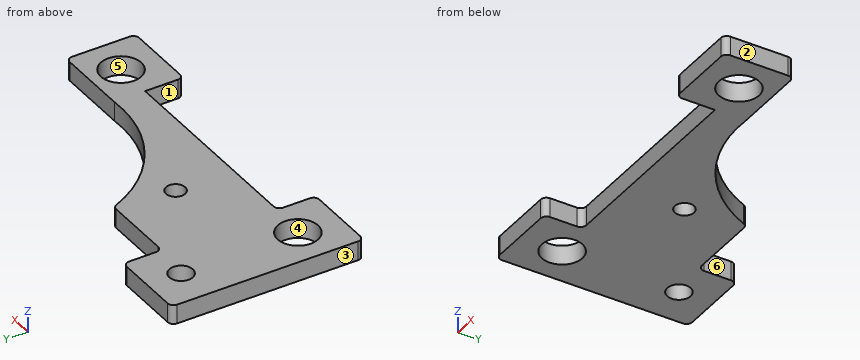
Autodesk Inventor part; units mm, degrees
ref_plane "YZ Plane" through (0, 0, 0) normal (1, 0, 0) x (0, 1, 0)
ref_plane "XZ Plane" through (0, 0, 0) normal (0, 1, 0) x (-1, 0, 0)
ref_plane "XY Plane" through (0, 0, 0) normal (0, 0, 1) x (1, 0, 0)
sketch "Esboço1" plane through (0, 0, 0) normal (0, 1, 0) x (-1, 0, 0)
  point P0 (0, 0)
sketch "Esboço2" plane through (0, 0, 0) normal (0, 0, 1) x (1, 0, 0)
  line L0 (0, 0) -> (20, 0)
  line L1 (20, 0) -> (20, 10)
  line L2 (20, 10) -> (75, 10)
  line L3 (75, 10) -> (75, 0)
  line L4 (75, 0) -> (95, 0)
  line L5 (95, 0) -> (95, 18)
  line L6 (95, 18) -> (75, 18)
  line L7 (0, 0) -> (0, 50)
  line L8 (0, 50) -> (20, 50)
  line L9 (20, 50) -> (20, 40)
  line L10 (20, 40) -> (40, 40)
  arc A0 (40, 40) -> (75, 18) centre (72.5309, 52.9128) ccw
  circle A1 centre (10, 41.2323) radius 3.05
  circle A2 centre (10, 10.8785) radius 5.25
  circle A3 centre (85, 10) radius 5.25
  circle A4 centre (38.286, 25) radius 2.5
  dimension "d0" = 20
  dimension "d1" = 10
  dimension "d2" = 55
  dimension "d3" = 10
  dimension "d4" = 20
  dimension "d5" = 18
  dimension "d6" = 20
  dimension "d7" = 50
  dimension "d8" = 20
  dimension "d9" = 10
  dimension "d10" = 20
  dimension "d11" = 35
  dimension "d12" = 6.1
  dimension "d13" = 10.5
  dimension "d14" = 10.5
  dimension "d15" = 5
extrude "Extrusão1" add sketch "Esboço2" along normal blind 5
fillet "Arredondamento1" radius 1.5 2 edges at (0, 50, 2.5) (20, 50, 2.5)
fillet "Arredondamento2" radius 1.5 8 edges at (20, 40, 2.5) (40, 40, 2.5) (95, 0, 2.5) (75, 0, 2.5) (20, 0, 2.5) (20, 10, 2.5) (95, 18, 2.5) (0, 0, 2.5)
properties part number "lateralCanhao"
Check sheet for the modelled part. Datum: model origin and axes. Units: mm. Face numbers are marked on the shaded views. A direction names the side the tool comes from. Round coordinates to 2 decimals unless told otherwise and drop trailing zeros. Order: outer loops, then holes, each group sorted by start corner. A loop starts at its lowest first (then second) coordinate and runs counter-clockwise, first axis right, second up.
(1) Go/stop test with flat-tipped pins: P1, Ø17, axis at x = 85, y = 10, coming from the -Z side; P2, Ø3, axis at x = 38.286, y = 25, coming from the +Z side; P3, Ø2.5, axis at x = 82, z = 1.5, coming from the +Y side; P4, Ø2.5, axis at x = 42, z = 1.5, coming from the -Y side. Record where each tip stops, or that it passes through.
(2) Draft check along X on the marked faces 3, 4, 5 and 6. Enter one of: pulls with the +X half, pulls with the -X half, needs draft (parallel to the pull), parting line crosses it, or undercut.
(3) Cross-section at B-B, the plane x = 85. Enter the section's corners in (y, z).
(4) Cross-section at D-D, the plane y = 25. Enter the section's corners in (x, z), and give its area (3 significant figures).
(5) Cross-section at C-C, the plane z = 2.1. Enter the section's corners in (x, y), and give its area (3 significant figures).
(6) Scan lines: probe 1 along Y at (x, z) = (10, 1.45); probe 2 along Y at (x, z) = (85, 3.3); probe 3 along X at (y, z) = (11.5, 4.55). Record each from-to range of solid material in increasing order.
(7) Cross-section at A-A, the plane x = 10. Enter the section's corners in (y, z), and give its area (3 significant figures).
(8) Access from +Z, -Z, +X, -X, +Y, -Y to the whole of each face (thin tool, end or side, straight path). Record for the marked faces 1 and 2.
Check sheet entries:
1. P1: stops at z = 0
1. P2: passes through
1. P3: stops at y = 18
1. P4: stops at y = 10
2. face 3: pulls with the -X half
2. face 4: undercut
2. face 5: undercut
2. face 6: pulls with the +X half
3. outline: (0, 0) - (4.75, 0) - (4.75, 5) - (0, 5) - close; (15.25, 0) - (18, 0) - (18, 5) - (15.25, 5) - close
4. outline: (0, 0) - (35.79, 0) - (35.79, 5) - (0, 5) - close; (40.79, 0) - (51.42, 0) - (51.42, 5) - (40.79, 5) - close
4. area: 232 mm2
5. outline: (0, 1.5) arc R1.5 ccw to (1.5, 0) - (18.5, 0) arc R1.5 ccw to (20, 1.5) - (20, 8.5) arc R1.5 cw to (21.5, 10) - (75, 10) - (75, 1.5) arc R1.5 ccw to (76.5, 0) - (93.5, 0) arc R1.5 ccw to (95, 1.5) - (95, 16.5) arc R1.5 ccw to (93.5, 18) - (75, 18) arc R35 cw to (40.38, 39.09) arc R1.5 ccw to (39, 40) - (21.5, 40) arc R1.5 cw to (20, 41.5) - (20, 48.5) arc R1.5 ccw to (18.5, 50) - (1.5, 50) arc R1.5 ccw to (0, 48.5) - close; hole circle Ø10.5 at (10, 10.88); hole circle Ø6.1 at (10, 41.23); hole circle Ø5 at (38.29, 25); hole circle Ø10.5 at (85, 10)
5. area: 2,210 mm2
6. probe 1: y = 0 to 5.63, 16.13 to 38.18, 44.28 to 50
6. probe 2: y = 0 to 4.75, 15.25 to 18
6. probe 3: x = 0 to 4.79, 15.21 to 79.97, 90.03 to 95
7. outline: (0, 0) - (5.63, 0) - (5.63, 5) - (0, 5) - close; (16.13, 0) - (38.18, 0) - (38.18, 5) - (16.13, 5) - close; (44.28, 0) - (50, 0) - (50, 5) - (44.28, 5) - close
7. area: 167 mm2
8. face 1: +Z, -Z, -Y
8. face 2: +Z, -Z, +X, +Y, -Y
